```python
from build123d import *

# Parameters (mm, degrees)
SKETCH1_R           = 70
BOSS_EXTRUDE1_DEPTH = 5


with BuildPart() as part:
    # Sketch1 → Boss-Extrude1 (new body)
    with BuildSketch(Plane(origin=(0, 0, 0), x_dir=(1, 0, 0), z_dir=(0, 1, 0))):
        with Locations(Location((0, 0, 0), (0, 0, 270))):
            Circle(SKETCH1_R)
        with BuildLine():
            Line((55.319824044, 23.231811546), (13.090169944, 9.510565163))
            Line((13.090169944, 9.510565163), (39.189531511, 45.43325456))
            ThreePointArc((39.189531511, 45.43325456), (48.541019662, 35.267115138), (55.319824044, 23.231811546))
        make_face(mode=Mode.SUBTRACT)
        with BuildLine():
            Line((-5, 15.388417687), (-31.099361567, 51.311107083))
            ThreePointArc((-31.099361567, 51.311107083), (-18.541019662, 57.063390978), (-5, 59.791303716))
            Line((-5, 59.791303716), (-5, 15.388417687))
        make_face(mode=Mode.SUBTRACT)
        with BuildLine():
            Line((5, 15.388417686), (31.099361567, 51.311107083))
            ThreePointArc((31.099361567, 51.311107083), (18.541019662, 57.063390978), (5, 59.791303716))
            Line((5, 59.791303716), (5, 15.388417686))
        make_face(mode=Mode.SUBTRACT)
        with BuildLine():
            Line((58.409993988, 13.721246383), (16.180339887, 0))
            Line((16.180339887, 0), (58.409993988, -13.721246382))
            ThreePointArc((58.409993988, -13.721246382), (60, 0), (58.409993988, 13.721246383))
        make_face(mode=Mode.SUBTRACT)
        with BuildLine():
            Line((39.189531511, -45.43325456), (13.090169944, -9.510565163))
            Line((13.090169944, -9.510565163), (55.319824045, -23.231811545))
            ThreePointArc((55.319824045, -23.231811545), (48.541019663, -35.267115137), (39.189531511, -45.43325456))
        make_face(mode=Mode.SUBTRACT)
        with BuildLine():
            Line((31.099361568, -51.311107083), (5, -15.388417685))
            Line((5, -15.388417685), (5, -59.791303716))
            ThreePointArc((5, -59.791303716), (18.541019663, -57.063390978), (31.099361568, -51.311107083))
        make_face(mode=Mode.SUBTRACT)
        with BuildLine():
            Line((-55.319824044, 23.231811546), (-13.090169944, 9.510565163))
            Line((-13.090169944, 9.510565163), (-39.189531511, 45.43325456))
            ThreePointArc((-39.189531511, 45.43325456), (-48.541019662, 35.267115138), (-55.319824044, 23.231811546))
        make_face(mode=Mode.SUBTRACT)
        with BuildLine():
            Line((-58.409993988, 13.721246383), (-16.180339888, 0))
            Line((-16.180339888, 0), (-58.409993988, -13.721246382))
            ThreePointArc((-58.409993988, -13.721246382), (-60, 0), (-58.409993988, 13.721246383))
        make_face(mode=Mode.SUBTRACT)
        with BuildLine():
            Line((-39.189531511, -45.43325456), (-13.090169944, -9.510565163))
            Line((-13.090169944, -9.510565163), (-55.319824045, -23.231811545))
            ThreePointArc((-55.319824045, -23.231811545), (-48.541019663, -35.267115137), (-39.189531511, -45.43325456))
        make_face(mode=Mode.SUBTRACT)
        with BuildLine():
            Line((-31.099361568, -51.311107083), (-5, -15.388417686))
            Line((-5, -15.388417686), (-5, -59.791303715))
            ThreePointArc((-5, -59.791303715), (-18.541019663, -57.063390978), (-31.099361568, -51.311107083))
        make_face(mode=Mode.SUBTRACT)
        with BuildLine():
            Line((-1.5, -2), (1.5, -2))
            ThreePointArc((1.5, -2), (2.5, 0), (1.5, 2))
            Line((1.5, 2), (-1.5, 2))
            ThreePointArc((-1.5, 2), (-2.5, 0), (-1.5, -2))
        make_face(mode=Mode.SUBTRACT)
    extrude(amount=BOSS_EXTRUDE1_DEPTH)


solid = part.part
```
Geometry: final body of the model. Coordinates: model frame, mm. Give positions to 0.01 mm unless a question says otherwise; leave off trailing zeros. Write each loop counter-clockwise with the first axis right and the second up, starting at its lowest first coordinate (ties: lowest second). Pieces come first, ordered by that corner, then holes.
1. Line query: probe 1 along Z at (x, y) = (44, 3); probe 2 along Z at (x, y) = (46, 2.3); probe 3 along X at (y, z) = (0.25, -27.5). Output: solid intervals per line, ascending.
2. Section query D-D, the plane x = 44. Return loops of the section in (y, z).
3. Section query C-C, the plane y = 4. Count the separate pieces of the cut face and the enclosed holes in it, then the cut area to 3 significant figures.
4. Section query B-B, the plane x = 26. Return loops of the section in (y, z), then the cut area to 3 significant figures.
5. Draft query along X for faces 1 (the cylindrical face through (-42.594, 2.465, -55.55)), 2 (the flat face through (5, 2, 37)), 3 (the flat face through (25.957, 2.465, -27.22)), 4 (the flat face through (1, 0, 15)). Return one class per face: released by +X, released by -X, zero draft, split by the parting line, or undercut.
6. Pin query (flat end, axial travel): P1, Ø2.5, axis at y = 2, z = -44, coming from the +X side; P2, Ø3, axis at y = 2.5, z = 2, coming from the +X side; P3, Ø2.5, axis at x = 0.5, y = 3, coming from the +Z side; P4, Ø2.5, axis at y = 1.5, z = -41, coming from the -X side. Return the tip coordinate at first contact, or that it passes through.
7. Section query A-A, the plane x = 11.5. Return loops of the section in (y, z), then the cut area to 3 significant figures.
Computed:
1. probe 1: z = -54.44 to -40.79, -19.55 to -9.04, 9.04 to 19.55, 40.79 to 54.44
1. probe 2: z = -52.76 to -38.52, -20.2 to -9.69, 9.69 to 20.2, 38.52 to 52.76
1. probe 3: x = -64.37 to -53.33, -26.16 to -13.8, -5 to 5, 13.8 to 26.16, 53.33 to 64.37
2. outline: (0, -54.44) - (5, -54.44) - (5, -40.79) - (0, -40.79) - close; (0, -19.55) - (5, -19.55) - (5, -9.04) - (0, -9.04) - close; (0, 9.04) - (5, 9.04) - (5, 19.55) - (0, 19.55) - close; (0, 40.79) - (5, 40.79) - (5, 54.44) - (0, 54.44) - close
3. separate pieces: 1
3. enclosed holes: 11
3. area: 9,290 mm2
4. outline: (0, -64.99) - (5, -64.99) - (5, -54.07) - (0, -54.07) - close; (0, -44.29) - (5, -44.29) - (5, -27.28) - (0, -27.28) - close; (0, -13.71) - (5, -13.71) - (5, -3.19) - (0, -3.19) - close; (0, 3.19) - (5, 3.19) - (5, 13.71) - (0, 13.71) - close; (0, 27.28) - (5, 27.28) - (5, 44.29) - (0, 44.29) - close; (0, 54.07) - (5, 54.07) - (5, 64.99) - (0, 64.99) - close
4. area: 384 mm2
5. face 1: split by the parting line
5. face 2: undercut
5. face 3: undercut
5. face 4: zero draft
6. P1: stops at x = 55.43
6. P2: stops at x = 70
6. P3: stops at z = 70
6. P4: stops at x = -57.62
7. outline: (0, -69.05) - (5, -69.05) - (5, -58.89) - (0, -58.89) - close; (0, -24.33) - (5, -24.33) - (5, 24.33) - (0, 24.33) - close; (0, 58.89) - (5, 58.89) - (5, 69.05) - (0, 69.05) - close
7. area: 345 mm2
